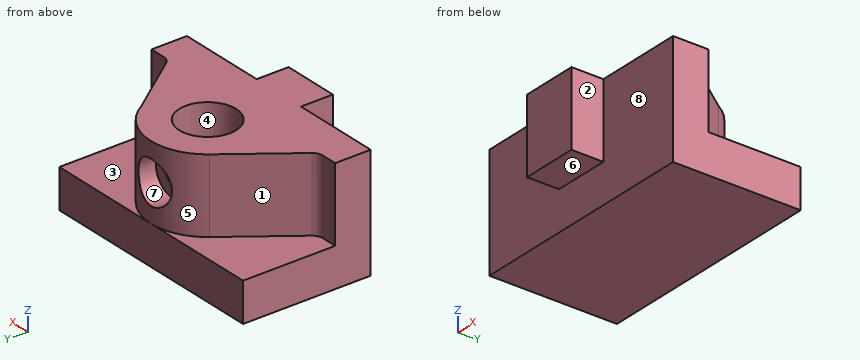
from build123d import *

# Parameters (mm, degrees)
SKETCH1_R              = 8
BOSS_EXTRUDE1_DEPTH    = 21
SKETCH2_W              = 66.3
SKETCH2_H              = 36
BOSS_EXTRUDE2_DEPTH    = 11
SKETCH19_R             = 6
CUT_EXTRUDE7_DEPTH     = 6
M6_TAPPED_HOLE1_REACH  = 57.517
M6_TAPPED_HOLE1_BORE_R = 2.5


with BuildPart() as part:
    # Sketch1 → Boss-Extrude1 (new body)
    with BuildSketch(Plane.XY):
        with BuildLine():
            Line((-33.15, -16), (-8, -16))
            Line((-8, -16), (-8, -25))
            Line((-8, -25), (8, -25))
            Line((8, -25), (8, -16))
            Line((8, -16), (33.15, -16))
            Line((33.15, -16), (33.15, -6))
            Line((33.15, -6), (28.687572119, -6))
            ThreePointArc((28.687572119, -6), (27.334939497, -5.677757455), (26.272890727, -4.78025666))
            Line((26.272890727, -4.78025666), (14.048740351, 11.800177564))
            ThreePointArc((14.048740351, 11.800177564), (1.086707772, 19.968226779), (-12.799429053, 13.494702186))
            Line((-12.799429053, 13.494702186), (-26.272890727, -4.78025666))
            ThreePointArc((-26.272890727, -4.78025666), (-27.334939497, -5.677757455), (-28.687572119, -6))
            Line((-28.687572119, -6), (-33.15, -6))
            Line((-33.15, -6), (-33.15, -16))
        make_face()
        with Locations(Location((0.078871705, 4, 0), (0, 0, 180))):
            Circle(SKETCH1_R, mode=Mode.SUBTRACT)
    extrude(amount=BOSS_EXTRUDE1_DEPTH)

    # Sketch2 → Boss-Extrude2 (add)
    with BuildSketch(Plane(origin=(0, 0, 0), x_dir=(-1, 0, 0), z_dir=(0, 0, -1))):
        with Locations((0, 2)):
            Rectangle(SKETCH2_W, SKETCH2_H)
    extrude(amount=BOSS_EXTRUDE2_DEPTH)

    # Sketch19 → Cut-Extrude7 (cut)
    with BuildSketch(Plane(origin=(0, 20, 0), x_dir=(1, 0, 0), z_dir=(0, 1, 0))):
        with Locations(Location((0, -10.5, 0), (0, 0, 270))):
            Circle(SKETCH19_R)
    extrude(amount=-CUT_EXTRUDE7_DEPTH, mode=Mode.SUBTRACT)

    # M6 Tapped Hole1 bore (on position points) → M6 Tapped Hole1 (cut, up to next)
    with BuildSketch(Plane(origin=(0, 14, 10.5), x_dir=(0, 0, 1), z_dir=(0, 1, 0)), mode=Mode.PRIVATE) as m6_tapped_hole1_sk1:
        Circle(M6_TAPPED_HOLE1_BORE_R)
    m6_tapped_hole1_tool1 = extrude(m6_tapped_hole1_sk1.sketch, amount=-M6_TAPPED_HOLE1_REACH, mode=Mode.PRIVATE) & part.part
    add(m6_tapped_hole1_tool1.solids().sort_by_distance((0, 14, 10.5))[0], mode=Mode.SUBTRACT)


solid = part.part
For this review, take the finished solid that the model builds, in its own axes (mm). Face numbers are marked on the shaded views. A direction names the side the tool comes from. Give positions to 0.01 mm unless a question says otherwise; leave off trailing zeros. Order: outer loops, then holes, each group sorted by start corner. A loop starts at its lowest first (then second) coordinate and runs counter-clockwise, first axis right, second up. Notation, with made-up numbers: M -21,11 L 10,11 A14 ccw 10,25 Z; hole C 2.25,-20 d7. An arc over 180 degrees is marked long. Answer in a Markdown table with one row per item. Add a question column.
(1) For the marked faces 1, 2, 3, 4 and 5, list the 3-axis set-ups (+Z, -Z, +X, -X, +Y, -Y) from which the entire face can be reached by the end or side of a thin tool; tool diameter is ignored.
(2) Wall thickness on probe 1 along X at (y, z) = (-17, 6); probe 2 along Y at (x, z) = (-4, 12); probe 3 along Y at (x, z) = (-11, -1): over which ranges is each line inside the solid? List them lowest first. Write a range as [from, to].
(3) Consider section D-D on z = 11. State the section outline as (x, y) points.
(4) Consider section A-A on z = 18. State the section outline as (x, y) points, and give its area (3 significant figures).
(5) For pin 1 (1.5 mm diameter, centred on y = 14, z = 11.5, fed in from +X); pin 2 (4.5 mm diameter, centred on y = -21.5, z = 10.5, fed in from +X); pin 3 (8 mm diameter, centred on y = 11.5, z = 12, fed in from +X), all flat-tipped, find the tip position at first contact; note any pin that passes through.
(6) Mouldability with a two-part tool opening along Z and no side actions: class the marked faces 6, 7 and 8 as +Z half, -Z half, draft (parallel to the pull), parting line (faces both ways), or undercut.
(7) Consider section C-C on x = 29.5. State the section outline as (y, z) points, and give its area (3 significant figures).
Evaluation:
| question | item | result |
|---|---|---|
| 1 | face 1 | +Z, -X, +Y |
| 1 | face 2 | +Z, -Z, +X, -Y |
| 1 | face 3 | +Z, +X, +Y |
| 1 | face 4 | +Z |
| 1 | face 5 | +Z, +Y |
| 2 | probe 1 | x = [-8, 8] |
| 2 | probe 2 | y = [-25, -2.88], [10.88, 14] |
| 2 | probe 3 | y = [-16, 20] |
| 3 | outline | M -33.15,-16 L -8,-16 L -8,-25 L 8,-25 L 8,-16 L 33.15,-16 L 33.15,-6 L 28.69,-6 A3 cw 26.27,-4.78 L 14.05,11.8 A16 ccw 5.98,18.87 L 5.98,14 L 2.45,14 L 2.45,11.64 A8 cw long -2.45,11.59 L -2.45,14 L -5.98,14 L -5.98,18.81 A16 ccw -12.8,13.49 L -26.27,-4.78 A3 cw -28.69,-6 L -33.15,-6 Z |
| 4 | outline | M -33.15,-16 L -8,-16 L -8,-25 L 8,-25 L 8,-16 L 33.15,-16 L 33.15,-6 L 28.69,-6 A3 cw 26.27,-4.78 L 14.05,11.8 A16 ccw -12.8,13.49 L -26.27,-4.78 A3 cw -28.69,-6 L -33.15,-6 Z; hole C 0.08,4 d16 |
| 4 | area | 1,500 mm^2 |
| 5 | pin 1 | stops at x = 13.13 |
| 5 | pin 2 | stops at x = 8 |
| 5 | pin 3 | stops at x = 17.22 |
| 6 | face 6 | -Z half |
| 6 | face 7 | undercut |
| 6 | face 8 | draft |
| 7 | outline | M -16,-11 L 20,-11 L 20,0 L -6,0 L -6,21 L -16,21 Z |
| 7 | area | 606 mm^2 |
